Can you work these out from the model? Positions are in its coordinate system, mm. Face numbers are marked on the shaded views. A direction names the side the tool comes from. Give positions to 0.01 mm unless a question says otherwise; leave off trailing zeros. Loops run counter-clockwise (first coordinate to the right, second up) from the corner with the lowest first, then second, coordinate; pieces in that order, holes last. Notation, with made-up numbers: (48.5, 46.25) -> (90.5, 46.25) arc R31 ccw to (90.5, 77.25) -> close; hole circle Ø6 at (41.5, -6). An arc over 180 degrees is marked (long way). Return JSON: item names as keys, results as strings. Group by question number.
Q1. Will these pins go through, and if not, where does the flat tip stop? pin 1 (1.1 mm diameter, centred on x = -5.5, z = 2.5, fed in from +Y); pin 2 (5.5 mm diameter, centred on x = -15.5, y = 11, fed in from -Z); pin 3 (5 mm diameter, centred on x = -8, z = 4, fed in from +Y).
Q2. Suppose I cut it at A-A, the plane y = 0. Please give me the cut outline in (x, z).
Q3. I need wall thicknesses on line 1 along X through (y, z) = (0, 2.75); line 2 along Y through (x, z) = (-11.15, 9); line 3 along X through (y, z) = (-3, 11.25). Which ranges of each line are inside material? Lowest first, please. Write a range as [from, to].
Q4. Suppose I cut it at D-D, the plane x = -17. Please give me the cut outline in (y, z), and give its area (3 significant figures).
Q5. Thinking about a two-plate mould opening in Y: for the marked faces 1, 2, 3 and 4, which applies, pulls with the +Y half, pulls with the -Y half, needs draft (parallel to the pull), parting line crosses it, or undercut?
Q6. Which directions (+Z, -Z, +X, -X, +Y, -Y) give clear straight access to the entire face, cutting with the end or side of a thin tool? Please do the marked faces 5, 6, 7 and 8.
Q7. Suppose I cut it at B-B, the plane z = 9. Please give me the cut outline in (x, y).
Q8. Suppose I cut it at C-C, the plane y = 15. Please give me the cut outline in (x, z), and give its area (3 significant figures).
```python
from build123d import *

# Parameters (mm, degrees)
BOSS_EXTRUDE1_DEPTH  = 18
BOSS_EXTRUDE2_START  = -49.083485
SKETCH2_W            = 9.5
SKETCH2_H            = 10
BOSS_EXTRUDE2_DEPTH  = 49.083485
M3_CLEARANCE_HOLE1_D = 3.1
BOSS_EXTRUDE3_DEPTH  = 1.5
CHAMFER1_SIZE        = 0.5
SKETCH8_W            = 5
SKETCH8_H            = 9.5
CUT_EXTRUDE1_DEPTH   = 56.463952257
SKETCH9_W            = 8
SKETCH9_H            = 8.5
BOSS_EXTRUDE4_DEPTH  = 15
SKETCH13_W           = 33.5
SKETCH13_H           = 18
CUT_EXTRUDE5_DEPTH   = 61.010415763
SKETCH10_R           = 1.55
CUT_EXTRUDE6_DEPTH   = 2.6
CHAMFER2_SIZE        = 0.5


with BuildPart() as part:
    # Sketch1 → Boss-Extrude1 (new body)
    with BuildSketch(Plane.XY):
        with BuildLine():
            Line((-0.916515139, 2), (-50, 2))
            Line((-50, 2), (-50, -2))
            Line((-50, -2), (-0.916515139, -2))
            ThreePointArc((-0.916515139, -2), (-2.2, 0), (-0.916515139, 2))
        make_face()
    extrude(amount=BOSS_EXTRUDE1_DEPTH)

    # Sketch2 → Boss-Extrude2 (add)
    with BuildSketch(Plane.ZY.offset(50).offset(BOSS_EXTRUDE2_START)):
        with Locations((9, 0)):
            Rectangle(SKETCH2_W, SKETCH2_H)
    extrude(amount=BOSS_EXTRUDE2_DEPTH)

    # M3 Clearance Hole1 (through all)
    with Locations(Plane.XY.offset(18)):
        with Locations((-10, 0)):
            Hole(M3_CLEARANCE_HOLE1_D / 2)

    # Sketch7 → Boss-Extrude3 (add)
    with BuildSketch(Plane.ZY.offset(50)):
        Polygon((0, 2), (0, -2), (4.25, -2), (4.25, -5), (13.75, -5), (13.75, -2), (18, -2), (18, 2), (13.75, 2), (13.75, 5), (4.25, 5), (4.25, 2), align=None)
    extrude(amount=BOSS_EXTRUDE3_DEPTH)

    # Chamfer1
    # the kernel refuses this chamfer: 0.5 mm, written as the material it takes off along each edge
    with BuildSketch(Plane(origin=(-52.785841494, -2, 18), x_dir=(0, 0.9996219169112968, 0.027495876610589075), z_dir=(1, 0, 0)), Plane(origin=(0.369326355, 2, 0), x_dir=(0, 0.027495876610586494, 0.9996219169112968), z_dir=(-1, 0, 0))) as chamfer1_piece_1:
        Polygon((CHAMFER1_SIZE * 0.999621916911, -CHAMFER1_SIZE * 0.0274958766106), (-CHAMFER1_SIZE * 0.0274958766106, -CHAMFER1_SIZE * 0.999621916911), (0, 0), align=None)
    extrude(amount=53.155167849, mode=Mode.SUBTRACT)
    with BuildSketch(Plane(origin=(0.369326494, -5, 4.25), x_dir=(0, -0.027495876610585647, 0.9996219169112968), z_dir=(-1, 0, 0)), Plane(origin=(-52.785841494, 5, 4.25), x_dir=(0, 0.027495876610585647, 0.9996219169112968), z_dir=(1, 0, 0)), Plane(origin=(0.369326494, -5, 13.75), x_dir=(0, 0.9996219169112968, 0.027495876610585647), z_dir=(-1, 0, 0))) as chamfer1_piece_2:
        Polygon((CHAMFER1_SIZE * 0.999621916911, CHAMFER1_SIZE * 0.0274958766106), (-CHAMFER1_SIZE * 0.0274958766106, CHAMFER1_SIZE * 0.999621916911), (0, 0), align=None)
    extrude(amount=53.155167988, mode=Mode.SUBTRACT)
    with BuildSketch(Plane(origin=(-52.785841494, 5, 13.75), x_dir=(0, 0.027495876610585647, -0.9996219169112968), z_dir=(1, 0, 0))) as chamfer1_piece_3:
        Polygon((CHAMFER1_SIZE * 0.999621916911, -CHAMFER1_SIZE * 0.0274958766106), (-CHAMFER1_SIZE * 0.0274958766106, -CHAMFER1_SIZE * 0.999621916911), (0, 0), align=None)
    extrude(amount=53.155167988, mode=Mode.SUBTRACT)
    with BuildSketch(Plane(origin=(0.369326355, -2, 0), x_dir=(0, -0.027495876610586494, 0.9996219169112968), z_dir=(-1, 0, 0)), Plane(origin=(0.369326355, 2, 18), x_dir=(0, 0.027495876610586414, -0.9996219169112968), z_dir=(-1, 0, 0))) as chamfer1_piece_4:
        Polygon((CHAMFER1_SIZE * 0.999621916911, CHAMFER1_SIZE * 0.0274958766106), (-CHAMFER1_SIZE * 0.0274958766106, CHAMFER1_SIZE * 0.999621916911), (0, 0), align=None)
    extrude(amount=53.155167849, mode=Mode.SUBTRACT)

    # Sketch8 → Cut-Extrude1 (cut, through all)
    with BuildSketch(Plane(origin=(0, 5, 0), x_dir=(1, 0, 0), z_dir=(0, 1, 0))):
        with Locations((-2.5, -9)):
            Rectangle(SKETCH8_W, SKETCH8_H)
    extrude(amount=-CUT_EXTRUDE1_DEPTH, mode=Mode.SUBTRACT)

    # Sketch9 → Boss-Extrude4 (add)
    with BuildSketch(Plane(origin=(0, 5, 0), x_dir=(1, 0, 0), z_dir=(0, 1, 0))):
        with Locations((-14, -9)):
            Rectangle(SKETCH9_W, SKETCH9_H)
    extrude(amount=BOSS_EXTRUDE4_DEPTH)

    # Sketch13 → Cut-Extrude5 (cut, through all)
    with BuildSketch(Plane(origin=(0, 20, 0), x_dir=(1, 0, 0), z_dir=(0, 1, 0))):
        with Locations((-34.75, -9)):
            Rectangle(SKETCH13_W, SKETCH13_H)
    extrude(amount=-CUT_EXTRUDE5_DEPTH, mode=Mode.SUBTRACT)

    # Sketch10 → Cut-Extrude6 (cut)
    with BuildSketch(Plane.ZY.offset(10)):
        with Locations((9, 15)):
            Circle(SKETCH10_R)
    extrude(amount=CUT_EXTRUDE6_DEPTH, mode=Mode.SUBTRACT)

    # Chamfer2
    chamfer2_edges = [part.edges().sort_by_distance(p)[0] for p in [
        (-5, -5, 9),
        (-5, 5, 9),
        (-10, 12.5, 13.25),
        (-10, 12.5, 4.75),
        (-18, 12.5, 4.75),
        (-18, 12.5, 13.25),
        (-10, 20, 9),
        (-14, 20, 4.75),
        (-18, 20, 9),
        (-14, 20, 13.25),
        (-18, -3.25, 4.25),
        (-18, -4.75, 4.5),
        (-18, -1.75, 0.25),
        (-18, -4.75, 13.5),
        (-18, -3.25, 13.75),
        (-18, -1.75, 17.75),
        (-18, 1.75, 0.25),
        (-18, 4.75, 4.5),
        (-18, 3.25, 4.25),
        (-18, 1.75, 17.75),
        (-18, 3.25, 13.75),
        (-18, 4.75, 13.5),
        (-18, 2, 15.625),
        (-18, -2, 15.625),
        (-18, -5, 9),
        (-18, -2, 2.375),
        (-18, 0, 0),
        (-18, 2, 2.375),
        (-18, 0, 18),
        (-10, 15, 7.45),
    ]]
    chamfer(chamfer2_edges, length=CHAMFER2_SIZE)


solid = part.part
```
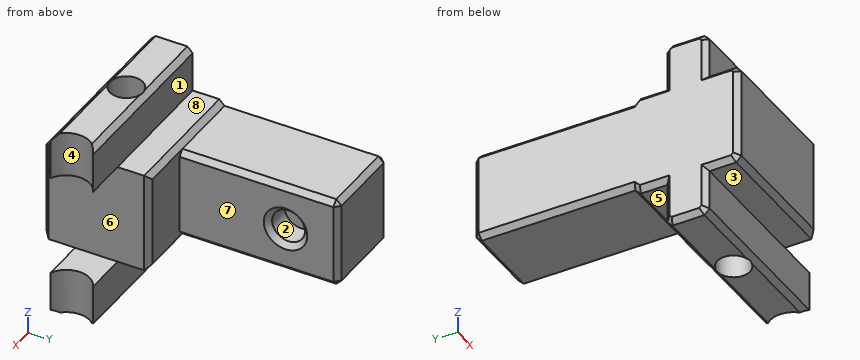
Ans:
{
 "1": {"pin 1": "stops at y = 2", "pin 2": "stops at z = 4.75", "pin 3": "stops at y = 19.67"},
 "2": {"outline": "(-18, 0.5) -> (-17.5, 0) -> (-11.55, 0) -> (-11.55, 18) -> (-17.5, 18) -> (-18, 17.5) -> close; (-8.45, 0) -> (-2.2, 0) -> (-2.2, 4.25) -> (-5, 4.25) -> (-5, 13.75) -> (-2.2, 13.75) -> (-2.2, 18) -> (-8.45, 18) -> close"},
 "3": {"line 1": "x = [-18, -11.55], [-8.45, -2.2]", "line 2": "y = [-5, -1.04], [1.04, 13.45], [16.55, 20]", "line 3": "x = [-18, -5]"},
 "4": {"outline": "(-5, 4.75) -> (-4.5, 4.25) -> (-2, 4.25) -> (-2, 0.5) -> (-1.5, 0) -> (1.5, 0) -> (2, 0.5) -> (2, 4.25) -> (4.5, 4.25) -> (5, 4.75) -> (19.5, 4.75) -> (20, 5.25) -> (20, 12.75) -> (19.5, 13.25) -> (5, 13.25) -> (4.5, 13.75) -> (2, 13.75) -> (2, 17.5) -> (1.5, 18) -> (-1.5, 18) -> (-2, 17.5) -> (-2, 13.75) -> (-4.5, 13.75) -> (-5, 13.25) -> close", "area": "255 mm^2"},
 "5": {"face 1": "pulls with the +Y half", "face 2": "undercut", "face 3": "needs draft", "face 4": "undercut"},
 "6": {"face 5": "-Z, +X, -X, +Y", "face 6": "+X, +Y, -Y", "face 7": "+Z, -Z, +X, +Y", "face 8": "+Z, +X, -X, +Y"},
 "7": {"outline": "(-18, -4.5) -> (-17.5, -5) -> (-5.5, -5) -> (-5, -4.5) -> (-5, 4.5) -> (-5.5, 5) -> (-10, 5) -> (-10, 12.95) -> (-10.5, 13.45) -> (-12.6, 13.45) -> (-12.6, 16.55) -> (-10.5, 16.55) -> (-10, 17.05) -> (-10, 19.5) -> (-10.5, 20) -> (-17.5, 20) -> (-18, 19.5) -> close; hole circle Ø3.1 at (-10, 0)"},
 "8": {"outline": "(-18, 5.25) -> (-17.5, 4.75) -> (-10.5, 4.75) -> (-10, 5.25) -> (-10, 6.95) -> (-10.5, 7.45) -> (-12.6, 7.45) -> (-12.6, 10.55) -> (-10.5, 10.55) -> (-10, 11.05) -> (-10, 12.75) -> (-10.5, 13.25) -> (-17.5, 13.25) -> (-18, 12.75) -> close", "area": "59.2 mm^2"}
}
